Autodesk Inventor part; units mm, degrees
ref_plane "YZ Plane" through (0, 0, 0) normal (1, 0, 0) x (0, 1, 0)
ref_plane "XZ Plane" through (0, 0, 0) normal (0, 1, 0) x (-1, 0, 0)
ref_plane "XY Plane" through (0, 0, 0) normal (0, 0, 1) x (1, 0, 0)
sketch "Sketch1" plane through (0, 0, 0) normal (0, 0, 1) x (1, 0, 0)
  line L0 (0, 0) -> (257.8074, 0)
  line L1 (275.5926, 25.4) -> (0, 25.4)
  line L2 (0, 25.4) -> (0, 0)
  line L3 (0, 12.7) -> (266.7, 12.7) construction
  line L4 (266.7, 12.7) -> (310.1366, -106.641) construction
  line L5 (275.5926, 25.4) -> (323.6516, -106.641)
  line L6 (323.6516, -106.641) -> (296.6215, -106.641)
  line L7 (296.6215, -106.641) -> (257.8074, 0)
  dimension "d4" = 25.4
  dimension "d5" = 110
  dimension "d6" = 266.7
  dimension "d7" = 127
  dimension "d17" = 110
  dimension "d18" = 25.4
extrude "Extrusion3" add sketch "Sketch1" along normal blind 25.4
shell "Shell3" thickness 1.5875 removed faces 2 at (0, 16.9333, 8.4667) at (305.6315, -106.641, 8.4667)
sketch "Sketch4" plane through (0, 0, 25.4) normal (0, 0, 1) x (1, 0, 0)
  line L0 (0, 0) -> (0, 25.4)
  line L1 (257.8074, 0) -> (0, 0)
  circle A0 centre (12.7, 12.7) radius 3.175
  dimension "d21" = 6.35
  dimension "d22" = 12.7
  dimension "d23" = 12.7
extrude "Extrusion4" cut sketch "Sketch4" against normal through all
fillet "Fillet2" radius 12.7 2 edges at (0, 0, 12.7) (0, 25.4, 12.7)
properties part number "UpperArm" material "Aluminum-6061"
CAD build for the part. Positions are in the model's coordinates, mm. A direction names the side the tool comes from. Round coordinates to 2 decimals unless told otherwise and drop trailing zeros. Write each loop counter-clockwise with the first axis right and the second up, starting at its lowest first coordinate (ties: lowest second). Pieces come first, ordered by that corner, then holes. Notation, with made-up numbers: M 74,-1 L 88,-1 A21 cw 88,10 Z; hole C 31,24.5 d10. An arc over 180 degrees is marked long. Use a Markdown table: item, result. Add a question column.
1. Pull direction X, two halves, no side cores. Call faces 5 (the face through (310, -106.641, 1)), 6 (the face through (299.286, -39.696, 12.522)), 7 (the face through (278.89, -53.28, 12.54)): released by +X, released by -X, zero draft, split by the parting line, or undercut.
2. Slice it at A-A on z = 20.5. Give the cut face in (x, y), then the cut area to 3 significant figures.
3. Flat gauge pins, fed straight in: P1, Ø7.5, axis at x = 105.5, z = 15.5, coming from the -Y side; P2, Ø5, axis at x = 12.7, y = 12.7, coming from the +Z side; P3, Ø1, axis at y = -74, z = 3, coming from the -X side; P4, Ø1.5, axis at y = -79, z = 12.5, coming from the +X side. Where does each tip first touch, or does it go through?
4. Slice it at C-C on y = 12.7. Give the cut face in (x, z) (1 decimal).
5. Drill centre lines: probe 1 along Y at (x, z) = (81, 19.25); probe 2 along Y at (x, z) = (12.7, 0.6) (3 decimals). Where is each one in solid material? Low to high.
6. 3-axis set-ups, long thin cutter, end or side, ignore diameter. For faces 1 (the face through (172, 2, 1.588)), 2 (the face through (10.77, 0.147, 9.7)), 3 (the face through (131, 1.588, 13)), 4 (the face through (134, 0, 13)): which of +Z, -Z, +X, -X, +Y, -Y reach the whole face in a straight line?
7. Slice it at D-D on y = -25.5. Give the cut face in (x, z), then the cut area to 3 significant figures.
8. Slice it at B-B on x = 201. Give the cut face in (y, z).
Reply:
| question | item | result |
|---|---|---|
| 1 | face 5 | zero draft |
| 1 | face 6 | released by +X |
| 1 | face 7 | undercut |
| 2 | outline | M 6.55,1.59 A12.7 ccw 12.7,0 L 257.81,0 L 296.62,-106.64 L 298.31,-106.64 L 258.92,1.59 Z; M 6.55,23.81 L 274.48,23.81 L 321.96,-106.64 L 323.65,-106.64 L 275.59,25.4 L 12.7,25.4 A12.7 ccw Z |
| 2 | area | 1,220 mm^2 |
| 3 | P1 | stops at y = 0 |
| 3 | P2 | passes through |
| 3 | P3 | stops at x = 284.56 |
| 3 | P4 | stops at x = 313.86 |
| 4 | outline | M 0,0 L 9.5,0 L 9.5,1.6 L 0,1.6 Z; M 0,23.8 L 9.5,23.8 L 9.5,25.4 L 0,25.4 Z; M 15.9,0 L 280.2,0 L 280.2,25.4 L 15.9,25.4 L 15.9,23.8 L 278.5,23.8 L 278.5,1.6 L 15.9,1.6 Z |
| 5 | probe 1 | y = 0 to 1.59, 23.81 to 25.4 |
| 5 | probe 2 | y = 0 to 9.525, 15.875 to 25.4 |
| 6 | face 1 | none |
| 6 | face 2 | +Z, -Z, -X |
| 6 | face 3 | -X |
| 6 | face 4 | +Z, -Z, -X, -Y |
| 7 | outline | M 267.09,0 L 294.12,0 L 294.12,25.4 L 267.09,25.4 Z; hole M 268.78,1.59 L 292.43,1.59 L 292.43,23.81 L 268.78,23.81 Z |
| 7 | area | 161 mm^2 |
| 8 | outline | M 0,0 L 25.4,0 L 25.4,25.4 L 0,25.4 Z; hole M 1.59,1.59 L 23.81,1.59 L 23.81,23.81 L 1.59,23.81 Z |
